The listing builds one solid part. Answer for the finished solid, in the listing's coordinates (mm). A direction names the side the tool comes from. Round coordinates to 2 decimals unless told otherwise and drop trailing zeros. Write each loop counter-clockwise with the first axis right and the second up, starting at its lowest first coordinate (ties: lowest second). Pieces come first, ordered by that corner, then holes. Notation, with made-up numbers: (8.25, 26) - (17.25, 26) arc R21 cw to (17.25, 50) - close; hole circle Ø3 at (56.5, 87.5). An arc over 180 degrees is marked (long way). Use a Markdown table: item, result. Add a question column.
1) A cutting plane is placed at D-D (y = -28). Give the vertices of the cut face in (x, z).
2) Determine the mould class of faces 4 (the cylindrical face through (0.036, 0.815, -0.726)), 5 (the flat face through (0.04, -8.78, 3.15)), 6 (the cylindrical face through (0.04, -0.55, 2.6)), 7 (the flat face through (0, -6, 5.08)) for opening direction Y: +Y half, -Y half, draft (parallel to the pull), parting line (faces both ways), or undercut.
3) A cutting plane is placed at C-C (z = 19). Give the vertices of the cut face in (x, y), then the cut area to 3 significant figures.
4) Find the intervals of material crossed by probe 1 along Y at (x, z) = (-0.05, 6.5); probe 2 along Z at (x, y) = (-2, -1.5); probe 3 along Z at (x, y) = (-1.35, 2), in increasing order. Write a range as from..to.
5) A cutting plane is placed at B-B (y = -0.5). Give the vertices of the cut face in (x, z), then the cut area to 3 significant figures.
6) A tool of negligible diameter and unlimited length cuts with its end or side. For faces 1 (the flat face through (0, 0, 25.4)), 2 (the flat face through (0.04, -34.18, 4.08)), 3 (the flat face through (0, -4.953, 15)), from which of +Z, -Z, +X, -X, +Y, -Y can it reach the whole face along a straight path? Write none if from no direction.
7) This flat-tipped pin is pushed along its axis until it touches: P1, Ø3, axis at x = 1, y = -6, coming from the +Z side. Where does it stop, or does it pass through?
```python
from build123d import *

# Parameters (mm, degrees)
F0_W      = 5.08
F0_H      = 9.906
F1_DEPTH  = 25.4
F2_W      = 5.08
F2_H      = 5.08
F3_DEPTH  = 5.08
F4_W      = 5.08
F4_H      = 5.08
F5_DEPTH  = 5.08
F6_DEPTH  = 5.08
F7_DEPTH  = 25.4
F9_DEPTH  = 5.081
F10_R     = 2.41299
F11_R     = 2.54
F12_DEPTH = 5.081
F13_R     = 0.762


# Not quite as in the source:
# - a fillet or chamfer is up to 0.001 mm smaller than in the source, because OpenCascade refuses the exact size


with BuildPart() as f1:
    # F0 (on Top) → F1 (new body)
    with BuildSketch(Plane.XY):
        Rectangle(F0_W, F0_H)
    extrude(amount=F1_DEPTH)

    # F2 (on face) → F3 (join)
    with BuildSketch(Plane.XZ.offset(4.953)):
        with Locations((0, 2.54)):
            Rectangle(F2_W, F2_H)
    extrude(amount=F3_DEPTH)

    # F4 (on face) → F5 (join)
    with BuildSketch(Plane(origin=(0, 0, 0), x_dir=(1, 0, 0), z_dir=(0, 0, -1))):
        with Locations((0, 7.493)):
            Rectangle(F4_W, F4_H)
    extrude(amount=F5_DEPTH)

    # F6 (add): a face of the model
    f6_faces = [f1.faces().sort_by_distance(p)[0] for p in [
        (0, -4.953, -2.54),
    ]]
    extrude(f6_faces, amount=F6_DEPTH)

    # F7 (add): a face of the model
    f7_faces = [f1.faces().sort_by_distance(p)[0] for p in [
        (0, -10.033, 0),
    ]]
    extrude(f7_faces, amount=F7_DEPTH)

    # F8 (on face) → F9 (cut, through all)
    with BuildSketch(Plane.YZ.offset(2.54)):
        Polygon((-7.493, 5.08), (-10.033, 5.08), (-10.033, 1.27), align=None)
        Polygon((-10.033, 5.08), (-12.573, 5.08), (-12.573, 1.468039654), (-10.033, 1.27), align=None)
        Polygon((-12.573, 5.08), (-15.113, 5.08), (-15.113, 1.6660793079), (-12.573, 1.468039654), align=None)
        Polygon((-15.113, 5.08), (-17.653, 5.08), (-17.653, 1.8641189619), (-15.113, 1.6660793079), align=None)
        Polygon((-20.193, 5.08), (-22.733, 5.08), (-22.733, 2.2601982699), (-20.193, 2.0621586159), align=None)
        Polygon((-17.653, 5.08), (-20.193, 5.08), (-20.193, 2.0621586159), (-17.653, 1.8641189619), align=None)
        Polygon((-22.733, 5.08), (-25.273, 5.08), (-25.273, 2.4582379238), (-22.733, 2.2601982699), align=None)
        Polygon((-25.273, 5.08), (-27.813, 5.08), (-27.813, 2.6562775778), (-25.273, 2.4582379238), align=None)
        Polygon((-27.813, 5.08), (-30.353, 5.08), (-30.353, 2.8543172318), (-27.813, 2.6562775778), align=None)
        Polygon((-30.353, 5.08), (-32.893, 5.08), (-32.893, 3.0523568857), (-30.353, 2.8543172318), align=None)
        Polygon((-32.893, 5.08), (-35.433, 5.08), (-32.893, 3.0523568857), align=None)
    extrude(amount=-F9_DEPTH, mode=Mode.SUBTRACT)

    # F10 (radius 2.413 in the source; OpenCascade refuses exactly that, so slightly less here)
    f10_edges = [f1.edges().sort_by_distance(p)[0] for p in [
        (0, 0.127, -5.08),
        (0, 0.127, 0),
        (0, 4.953, 0),
    ]]
    fillet(f10_edges, radius=F10_R)

    # F11 (on face) → F12 (cut, through all)
    with BuildSketch(Plane.YZ.offset(2.54)):
        with Locations((0, 5.08)):
            Circle(F11_R)
    extrude(amount=-F12_DEPTH, mode=Mode.SUBTRACT)

    # F13
    f13_edges = [f1.edges().sort_by_distance(p)[0] for p in [
        (0, 4.953, 25.4),
        (0, -4.953, 25.4),
    ]]
    fillet(f13_edges, radius=F13_R)


solid = f1.part
```
Entries:
| question | item | result |
|---|---|---|
| 1 | outline | (-2.54, -5.08) - (2.54, -5.08) - (2.54, 2.67) - (-2.54, 2.67) - close |
| 2 | face 4 | +Y half |
| 2 | face 5 | undercut |
| 2 | face 6 | undercut |
| 2 | face 7 | draft |
| 3 | outline | (-2.54, -4.95) - (2.54, -4.95) - (2.54, 4.95) - (-2.54, 4.95) - close |
| 3 | area | 50.3 mm² |
| 4 | probe 1 | y = -4.95..-2.11, 2.11..4.95 |
| 4 | probe 2 | z = -4.95..3.03, 7.13..25.4 |
| 4 | probe 3 | z = -0.06..3.51, 6.65..25.4 |
| 5 | outline | (-2.54, -4.29) - (2.54, -4.29) - (2.54, 2.59) - (-2.54, 2.59) - close; (-2.54, 7.57) - (2.54, 7.57) - (2.54, 25.4) - (-2.54, 25.4) - close |
| 5 | area | 126 mm² |
| 6 | face 1 | +Z, +X, -X, +Y, -Y |
| 6 | face 2 | +Z, +X, -X |
| 6 | face 3 | +Z, +X, -X, -Y |
| 7 | P1 | stops at z = 25.33 |
